Could you check a few things on this model? Use its own coordinates, in mm. A direction names the side the tool comes from. Round coordinates to 2 decimals unless told otherwise and drop trailing zeros. Loops run counter-clockwise (first coordinate to the right, second up) from the corner with the lowest first, then second, coordinate; pieces in that order, holes last. Notation, with made-up numbers: (58, 71) -> (63, 71) arc R21 cw to (63, 96) -> close; hole circle Ø11 at (75, 61). An arc over 180 degrees is marked (long way). One line per item, written item: value.
from build123d import *

# Parameters (mm, degrees)
SALIENTE_EXTRUIR1_DEPTH                       = 50
CHAFL_N2_SIZE                                 = 3
CBORE_FOR_M2_HEX_HEAD_MACHINE_SCREW1_AT_COUNT = 2
CBORE_FOR_M2_HEX_HEAD_MACHINE_SCREW1_AT_PITCH = 12
CBORE_FOR_M2_HEX_HEAD_MACHINE_SCREW1_2_COUNT  = 2
CBORE_FOR_M2_HEX_HEAD_MACHINE_SCREW1_2_PITCH  = 23.40961341
CBORE_FOR_M2_HEX_HEAD_MACHINE_SCREW1_3_COUNT  = 2
CBORE_FOR_M2_HEX_HEAD_MACHINE_SCREW1_3_PITCH  = 20.1
CBORE_FOR_M2_HEX_HEAD_MACHINE_SCREW1_4_COUNT  = 2
CBORE_FOR_M2_HEX_HEAD_MACHINE_SCREW1_4_PITCH  = 28
CBORE_FOR_M2_HEX_HEAD_MACHINE_SCREW1_5_COUNT  = 2
CBORE_FOR_M2_HEX_HEAD_MACHINE_SCREW1_5_PITCH  = 34.467520944
CBORE_FOR_M2_HEX_HEAD_MACHINE_SCREW1_6_COUNT  = 2
CBORE_FOR_M2_HEX_HEAD_MACHINE_SCREW1_6_PITCH  = 44.766170263
CBORE_FOR_M2_HEX_HEAD_MACHINE_SCREW1_7_COUNT  = 2
CBORE_FOR_M2_HEX_HEAD_MACHINE_SCREW1_7_PITCH  = 40


with BuildPart() as part:
    # Croquis1 → Saliente-Extruir1 (new body)
    with BuildSketch(Plane.XY):
        with BuildLine():
            Line((0, 0), (8, 0))
            ThreePointArc((8, 0), (14.05, 3.068493182), (20.1, 0))
            Line((20.1, 0), (28.1, 0))
            Line((28.1, 0), (28.1, 5))
            Line((28.1, 5), (0, 5))
            Line((0, 5), (0, 0))
        make_face()
    extrude(amount=SALIENTE_EXTRUIR1_DEPTH)

    # Chaflán2
    chafl_n2_edges = [part.edges().sort_by_distance(p)[0] for p in [
        (0, 5, 25),
        (28.1, 5, 25),
    ]]
    chamfer(chafl_n2_edges, length=CHAFL_N2_SIZE)

    # Croquis3 → CBORE for M2 Hex Head Machine Screw1 (revolve, cut)
    with BuildSketch(Plane(origin=(4, 5, 5), x_dir=(0, 0, 1), z_dir=(1, 0, 0))):
        Polygon((0, 0), (0, 7), (1.2, 6.278967257), (1.2, 1.6), (3.19, 1.6), (3.19, 0.025), (3.215, 0), align=None)
    cbore_for_m2_hex_head_machine_screw1 = revolve(axis=Axis((4, 11.35, 5), (0, -1, 0)), mode=Mode.SUBTRACT)

    # CBORE for M2 Hex Head Machine Screw1 at: CBORE for M2 Hex Head Machine Screw1 ×2
    with Locations(*[(0, 0, i * CBORE_FOR_M2_HEX_HEAD_MACHINE_SCREW1_AT_PITCH) for i in range(1, CBORE_FOR_M2_HEX_HEAD_MACHINE_SCREW1_AT_COUNT)]):
        add(cbore_for_m2_hex_head_machine_screw1, mode=Mode.SUBTRACT)

    # CBORE for M2 Hex Head Machine Screw1 2: CBORE for M2 Hex Head Machine Screw1 ×2
    with Locations(*[Vector(0.8586216119022935, 0, 0.5126099175535989) * (i * CBORE_FOR_M2_HEX_HEAD_MACHINE_SCREW1_2_PITCH) for i in range(1, CBORE_FOR_M2_HEX_HEAD_MACHINE_SCREW1_2_COUNT)]):
        add(cbore_for_m2_hex_head_machine_screw1, mode=Mode.SUBTRACT)

    # CBORE for M2 Hex Head Machine Screw1 3: CBORE for M2 Hex Head Machine Screw1 ×2
    with Locations(*[(i * CBORE_FOR_M2_HEX_HEAD_MACHINE_SCREW1_3_PITCH, 0, 0) for i in range(1, CBORE_FOR_M2_HEX_HEAD_MACHINE_SCREW1_3_COUNT)]):
        add(cbore_for_m2_hex_head_machine_screw1, mode=Mode.SUBTRACT)

    # CBORE for M2 Hex Head Machine Screw1 4: CBORE for M2 Hex Head Machine Screw1 ×2
    with Locations(*[(0, 0, i * CBORE_FOR_M2_HEX_HEAD_MACHINE_SCREW1_4_PITCH) for i in range(1, CBORE_FOR_M2_HEX_HEAD_MACHINE_SCREW1_4_COUNT)]):
        add(cbore_for_m2_hex_head_machine_screw1, mode=Mode.SUBTRACT)

    # CBORE for M2 Hex Head Machine Screw1 5: CBORE for M2 Hex Head Machine Screw1 ×2
    with Locations(*[Vector(0.5831576930893619, 0, 0.8123589754478582) * (i * CBORE_FOR_M2_HEX_HEAD_MACHINE_SCREW1_5_PITCH) for i in range(1, CBORE_FOR_M2_HEX_HEAD_MACHINE_SCREW1_5_COUNT)]):
        add(cbore_for_m2_hex_head_machine_screw1, mode=Mode.SUBTRACT)

    # CBORE for M2 Hex Head Machine Screw1 6: CBORE for M2 Hex Head Machine Screw1 ×2
    with Locations(*[Vector(0.44899976660931423, 0, 0.8935318738493784) * (i * CBORE_FOR_M2_HEX_HEAD_MACHINE_SCREW1_6_PITCH) for i in range(1, CBORE_FOR_M2_HEX_HEAD_MACHINE_SCREW1_6_COUNT)]):
        add(cbore_for_m2_hex_head_machine_screw1, mode=Mode.SUBTRACT)

    # CBORE for M2 Hex Head Machine Screw1 7: CBORE for M2 Hex Head Machine Screw1 ×2
    with Locations(*[(0, 0, i * CBORE_FOR_M2_HEX_HEAD_MACHINE_SCREW1_7_PITCH) for i in range(1, CBORE_FOR_M2_HEX_HEAD_MACHINE_SCREW1_7_COUNT)]):
        add(cbore_for_m2_hex_head_machine_screw1, mode=Mode.SUBTRACT)


solid = part.part
(1) If I drill on L1, parallel to Z at x = 4, y = 1.5; L2, parallel to Z at x = 4, y = 4.3; L3, parallel to X at y = 1.9, z = 45, over which ranges is the centre line in solid material (lowest first)?
Recorded:
L1: 0 to 3.8, 6.2 to 15.8, 18.2 to 31.8, 34.2 to 43.8, 46.2 to 50
L2: 0 to 1.81, 8.19 to 13.81, 20.19 to 29.81, 36.19 to 41.81, 48.19 to 50
L3: 0 to 2.8, 5.2 to 10.03, 18.07 to 22.9, 25.3 to 28.1
(2) I'm going to push flat-ended pins straight in: pin 1 Ø4 at (x, z) = (4, 45) entering from +Y; pin 2 Ø2 at (y, z) = (4, 5.5) entering from +X. Where does each tip first touch, or does it pass through?
Recorded:
pin 1: y = 3.4
pin 2: x = 27.1
(3) If we section it at B-B, the plane z = 10: Please give me the cut outline in (x, y).
Recorded:
outline: (0, 0) -> (8, 0) arc R7.5 cw to (20.1, 0) -> (28.1, 0) -> (28.1, 2) -> (25.1, 5) -> (3, 5) -> (0, 2) -> close
(4) If we section it at D-D, the plane y = 4.35: Please give me the cut outline in (x, z).
Recorded:
outline: (2.35, 0) -> (25.75, 0) -> (25.75, 2.27) arc R3.19 cw (long way) to (25.75, 7.73) -> (25.75, 14.27) arc R3.19 cw (long way) to (25.75, 19.73) -> (25.75, 30.27) arc R3.19 cw (long way) to (25.75, 35.73) -> (25.75, 42.27) arc R3.19 cw (long way) to (25.75, 47.73) -> (25.75, 50) -> (2.35, 50) -> (2.35, 47.73) arc R3.19 cw (long way) to (2.35, 42.27) -> (2.35, 35.73) arc R3.19 cw (long way) to (2.35, 30.27) -> (2.35, 19.73) arc R3.19 cw (long way) to (2.35, 14.27) -> (2.35, 7.73) arc R3.19 cw (long way) to (2.35, 2.27) -> close
(5) For faces 1 (the face through (23, 3.4, 6)), 2 (the face through (0, 1, 25)), which set-ups out of +Z, -Z, +X, -X, +Y, -Y let a thin tool reach every point of the face, with its end or its side?
Recorded:
face 1: +Y
face 2: +Z, -Z, -X, +Y, -Y
(6) If we section it at A-A, the plane z = 5: Give the number of separate pieces and of enclosed holes in the cut face, then the cut area to 3 significant figures.
Recorded:
separate pieces: 3
enclosed holes: 0
area: 73.2 mm²
(7) Thinking about a two-plate mould opening in X: for faces 3 (the face through (4.46, 1.72, 46.11)), 4 (the face through (7.19, 4.2, 32.89)), 5 (the face through (4, 0, 25)), 6 (the face through (26.9, 3.2, 24.7)), which applies, released by +X, released by -X, zero draft, split by the parting line, or undercut?
Recorded:
face 3: undercut
face 4: undercut
face 5: zero draft
face 6: released by +X
